```python
from build123d import *

# Parameters (mm, degrees)
F0_R     = 1.5
F1_DEPTH = 6


with BuildPart() as f1:
    # F0 (on Top) → F1 (new body)
    with BuildSketch(Plane.XY):
        Polygon((-20.092445, 11.328948), (-34.234581, 25.471083), (-44.234581, 15.471083), (-30.092445, 1.328948), (-44.234581, -12.813188), (-34.234581, -22.813188), (-20.092445, -8.671052), (19.907555, -8.671052), (19.907555, 11.328948), align=None)
        with Locations((-34.234629, -12.813236)):
            Circle(F0_R, mode=Mode.SUBTRACT)
        with Locations((-3.092445, -4.671052)):
            Circle(F0_R, mode=Mode.SUBTRACT)
        with Locations((-34.234629, 15.471131)):
            Circle(F0_R, mode=Mode.SUBTRACT)
        with Locations((-3.092445, 7.328948)):
            Circle(F0_R, mode=Mode.SUBTRACT)
        with Locations((9.907555, 1.328948)):
            Circle(F0_R, mode=Mode.SUBTRACT)
    extrude(amount=F1_DEPTH)


solid = f1.part
```
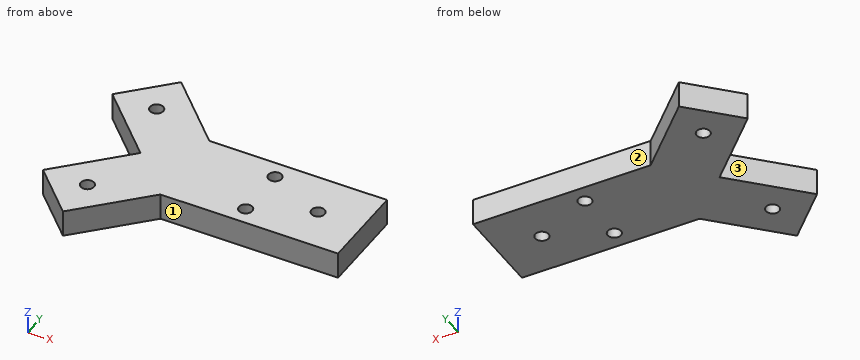
Input: part model. Units: mm. Frame: model coordinates. Face numbers are marked on the shaded views. A direction names the side the tool comes from. Give positions to 0.01 mm unless a question says otherwise; leave off trailing zeros. Order: outer loops, then holes, each group sorted by start corner. A loop starts at its lowest first (then second) coordinate and runs counter-clockwise, first axis right, second up. Notation, with made-up numbers: (72.5, 8) - (81.5, 8) arc R36 ccw to (81.5, 43) - close; hole circle Ø8 at (-23, 11.25). An arc over 180 degrees is marked (long way). Use a Markdown table: item, result.
(1) Section query D-D (y = -7). Output: boundary loops of the cut face in (x, z).
Computed values:
| item | result |
|---|---|
| outline | (-38.42, 0) - (19.91, 0) - (19.91, 6) - (-38.42, 6) - close |
(2) Section query A-A (x = -32). Output: boundary loops of the cut face in (y, z), then the cut area to 3 significant figures.
Computed values:
| item | result |
|---|---|
| outline | (-20.58, 0) - (-0.58, 0) - (-0.58, 6) - (-20.58, 6) - close; (3.24, 0) - (23.24, 0) - (23.24, 6) - (3.24, 6) - close |
| area | 240 mm2 |
(3) Section query C-C (z = 2.2). Output: boundary loops of the cut face in (x, y).
Computed values:
| item | result |
|---|---|
| outline | (-44.23, -12.81) - (-34.23, -22.81) - (-20.09, -8.67) - (19.91, -8.67) - (19.91, 11.33) - (-20.09, 11.33) - (-34.23, 25.47) - (-44.23, 15.47) - (-30.09, 1.33) - close; hole circle Ø3 at (-34.23, -12.81); hole circle Ø3 at (-34.23, 15.47); hole circle Ø3 at (-3.09, -4.67); hole circle Ø3 at (-3.09, 7.33); hole circle Ø3 at (9.91, 1.33) |
(4) Pin query (flat end, axial travel): pin 1 (1.8 mm diameter, centred on x = -1.5, z = 4, fed in from +Y); pin 2 (3 mm diameter, centred on x = -21, z = 1, fed in from -Y); pin 3 (2 mm diameter, centred on y = -8.5, z = 2, fed in from -X). Return the tip coordinate at first contact, or that it passes through.
Computed values:
| item | result |
|---|---|
| pin 1 | stops at y = 11.33 |
| pin 2 | stops at y = -11.08 |
| pin 3 | stops at x = -40.92 |
(5) Section query B-B (y = 0.5). Output: boundary loops of the cut face in (x, z), then the cut area to 3 significant figures.
Computed values:
| item | result |
|---|---|
| outline | (-30.92, 0) - (8.66, 0) - (8.66, 6) - (-30.92, 6) - close; (11.16, 0) - (19.91, 0) - (19.91, 6) - (11.16, 6) - close |
| area | 290 mm2 |
(6) Access query for the marked faces 1, 2 and 3. Directions: +Z, -Z, +X, -X, +Y, -Y. A direction counts if a zero-diameter tool reaches every point of the face in a straight line with its end or side. Return the directions, or none.
Computed values:
| item | result |
|---|---|
| face 1 | +Z, -Z, +X, -Y |
| face 2 | +Z, -Z, +X, +Y |
| face 3 | +Z, -Z, -X |
(7) Line query: line 1 (Y direction, x = 10, z = 5.7); line 2 (Y direction, x = -35, z = 4.2); line 3 (X direction, y = -12, z = 1.05). Output: solid intervals per line, ascending. Write a range as from..to.
Computed values:
| item | result |
|---|---|
| line 1 | y = -8.67..-0.17, 2.83..11.33 |
| line 2 | y = -22.05..-14.1, -11.52..-3.58, 6.24..14.18, 16.76..24.71 |
| line 3 | x = -43.42..-35.5, -32.97..-23.42 |
